Here's how the part is built. I have some questions about the finished solid (model axes, mm). Round coordinates to 2 decimals unless told otherwise and drop trailing zeros. Loops run counter-clockwise (first coordinate to the right, second up) from the corner with the lowest first, then second, coordinate; pieces in that order, holes last. Notation, with made-up numbers: (69, -35) -> (78, -35) arc R14 cw to (78, -17) -> close; hole circle Ø4 at (48.25, 31.25). An arc over 180 degrees is marked (long way). One line per item, written item: value. Start each with the question number.
```python
from build123d import *

# Parameters (mm, degrees)
SKETCH1_R           = 2.25
SKETCH1_R_2         = 2.75
BOSS_EXTRUDE1_DEPTH = 3.2


with BuildPart() as part:
    # Sketch1 → Boss-Extrude1 (new body)
    with BuildSketch(Plane.XY):
        with BuildLine():
            Line((5, 0), (405, 0))
            ThreePointArc((405, 0), (408.535533906, 1.464466094), (410, 5))
            Line((410, 5), (410, 295))
            ThreePointArc((410, 295), (408.535533906, 298.535533906), (405, 300))
            Line((405, 300), (5, 300))
            ThreePointArc((5, 300), (1.464466094, 298.535533906), (0, 295))
            Line((0, 295), (0, 5))
            ThreePointArc((0, 5), (1.464466094, 1.464466094), (5, 0))
        make_face()
        with Locations((310, 23.339430176)):
            Circle(SKETCH1_R, mode=Mode.SUBTRACT)
        with Locations((350, 23.156887411)):
            Circle(SKETCH1_R, mode=Mode.SUBTRACT)
        with Locations((390, 22.974344646)):
            Circle(SKETCH1_R, mode=Mode.SUBTRACT)
        with Locations((310, 137.974344646)):
            Circle(SKETCH1_R, mode=Mode.SUBTRACT)
        with Locations((350, 137.974344646)):
            Circle(SKETCH1_R, mode=Mode.SUBTRACT)
        with Locations((390, 137.974344646)):
            Circle(SKETCH1_R, mode=Mode.SUBTRACT)
        with Locations((300, 106)):
            Circle(SKETCH1_R_2, mode=Mode.SUBTRACT)
        with Locations((38.17, 106)):
            Circle(SKETCH1_R_2, mode=Mode.SUBTRACT)
        with Locations((38.17, 212)):
            Circle(SKETCH1_R_2, mode=Mode.SUBTRACT)
        with Locations((300, 212)):
            Circle(SKETCH1_R_2, mode=Mode.SUBTRACT)
        with BuildLine():
            Line((33, 155), (377, 155))
            ThreePointArc((377, 155), (379.121320344, 155.878679656), (380, 158))
            Line((380, 158), (380, 172))
            ThreePointArc((380, 172), (379.121320344, 174.121320344), (377, 175))
            Line((377, 175), (33, 175))
            ThreePointArc((33, 175), (30.878679656, 174.121320344), (30, 172))
            Line((30, 172), (30, 158))
            ThreePointArc((30, 158), (30.878679656, 155.878679656), (33, 155))
        make_face(mode=Mode.SUBTRACT)
    extrude(amount=BOSS_EXTRUDE1_DEPTH)


solid = part.part
```
Q1. I want a section at A-A on x = 209. Please give me the cut outline in (y, z).
Q2. I want a section at B-B on z = 1.3. State how many separate pieces and enclosed holes the cut face has, plus the area to 3 significant figures.
Q3. Will this pin go through, and if not, where does the flat tip stop? P1, Ø6.5, axis at x = 300, y = 106, coming from the -Z side.
Q4. If I drill on line 1 along Y through (x, z) = (390, 0.8); line 2 along Y through (x, z) = (350, 1.95); line 3 along X through (y, z) = (212, 1.4), over which ranges is the centre line in solid material (lowest first)?
Answers below:
1. outline: (0, 0) -> (155, 0) -> (155, 3.2) -> (0, 3.2) -> close; (175, 0) -> (300, 0) -> (300, 3.2) -> (175, 3.2) -> close
2. separate pieces: 1
2. enclosed holes: 11
2. area: 116,000 mm^2
3. P1: stops at z = 0
4. line 1: y = 0 to 20.72, 25.22 to 135.72, 140.22 to 300
4. line 2: y = 0 to 20.91, 25.41 to 135.72, 140.22 to 155, 175 to 300
4. line 3: x = 0 to 35.42, 40.92 to 297.25, 302.75 to 410
